Work out the finished part from the listing and answer in its coordinate system (mm). Coordinates: 2 decimals unless noted, no trailing zeros. Loops run counter-clockwise (first coordinate to the right, second up) from the corner with the lowest first, then second, coordinate; pieces in that order, holes last. Notation, with made-up numbers: (1, 15.5) -> (49, 15.5) arc R21 ccw to (49, 40.5) -> close; hole circle Ø11 at (19, -24). An arc over 180 degrees is marked (long way). One line per question, with ' | ' between items.
```python
from build123d import *

# Parameters (mm, degrees)
SKETCH1_R           = 1.5
BOSS_EXTRUDE1_DEPTH = 125


with BuildPart() as part:
    # Sketch1 → Boss-Extrude1 (new body)
    with BuildSketch(Plane(origin=(0, 0, 0), x_dir=(1, 0, 0), z_dir=(0, 1, 0))):
        with BuildLine():
            ThreePointArc((-3.151258993, -1.464647316), (-2.457196065, -2.457196065), (-1.464647316, -3.151258993))
            ThreePointArc((-1.464647316, -3.151258993), (0, -1.975), (1.464647316, -3.151258993))
            ThreePointArc((1.464647316, -3.151258993), (2.457196065, -2.457196065), (3.151258993, -1.464647316))
            ThreePointArc((3.151258993, -1.464647316), (1.975, 0), (3.151258993, 1.464647316))
            ThreePointArc((3.151258993, 1.464647316), (2.457196065, 2.457196065), (1.464647316, 3.151258993))
            ThreePointArc((1.464647316, 3.151258993), (0, 1.975), (-1.464647316, 3.151258993))
            ThreePointArc((-1.464647316, 3.151258993), (-2.457196065, 2.457196065), (-3.151258993, 1.464647316))
            ThreePointArc((-3.151258993, 1.464647316), (-1.975, 0), (-3.151258993, -1.464647316))
        make_face()
        with Locations(Location((0, 0, 0), (0, 0, 270))):
            Circle(SKETCH1_R, mode=Mode.SUBTRACT)
    extrude(amount=BOSS_EXTRUDE1_DEPTH)


solid = part.part
```
1) Find section A-A (x = 0). Write down the section's boundary in (y, z) (3 decimals), plus the area to 3 significant figures.
Check values:
outline: (0, -1.975) -> (125, -1.975) -> (125, -1.5) -> (0, -1.5) -> close; (0, 1.5) -> (125, 1.5) -> (125, 1.975) -> (0, 1.975) -> close | area: 119 mm^2
2) Find section C-C (z = 0). Write down the section's boundary in (x, y) (3 decimals).
Check values:
outline: (-1.975, 0) -> (-1.5, 0) -> (-1.5, 125) -> (-1.975, 125) -> close; (1.5, 0) -> (1.975, 0) -> (1.975, 125) -> (1.5, 125) -> close
3) Flat-ended cylindrical pins translate along their axes: pin 1 (2 mm diameter, centred on x = -2, y = 67, fed in from +Z); pin 2 (2 mm diameter, centred on x = 1.5, y = 107, fed in from -Z). Find the tip coordinate at first contact, or state that the pin passes through.
Check values:
pin 1: stops at z = 3.15 | pin 2: stops at z = -3.15
4) Find the intervals of material crossed by line 1 along X through (y, z) = (83, -0.25); line 2 along X through (y, z) = (59, -2.5); line 3 along Z through (x, y) = (-2.25, 117), in increasing order.
Check values:
line 1: x = -2 to -1.48, 1.48 to 2 | line 2: x = -2.41 to -1.14, 1.14 to 2.41 | line 3: z = -2.65 to -0.87, 0.87 to 2.65
5) Find section B-B (y = 91). Write down the section's boundary in (x, z) (3 decimals), plus the area to 3 significant figures.
Check values:
outline: (-3.151, -1.465) arc R3.475 ccw to (-1.465, -3.151) arc R1.5 cw to (1.465, -3.151) arc R3.475 ccw to (3.151, -1.465) arc R1.5 cw to (3.151, 1.465) arc R3.475 ccw to (1.465, 3.151) arc R1.5 cw to (-1.465, 3.151) arc R3.475 ccw to (-3.151, 1.465) arc R1.5 cw to start; hole circle Ø3 at (0, 0) | area: 18.0 mm^2
6) The mould has two halves that part along Z. Classify faces 1 (the face through (0.028, 61.625, -1.975)), 2 (the face through (1.975, 61.625, 0.028)), 3 (the face through (-0.028, 61.625, 1.975)): released by +Z, released by -Z, zero draft, split by the parting line, or undercut.
Check values:
face 1: released by -Z | face 2: undercut | face 3: released by +Z
